```python
from build123d import *

# Parameters (mm, degrees)
BOSS_EXTRUDE1_DEPTH   = 25.4
CUT_EXTRUDE1_REACH    = 329.931
F_8_CLEARANCE_HOLE1_D = 4.9149
CHAMFER1_SIZE         = 1.275307785
CHAMFER1_SIZE_2       = 1.27
CHAMFER1_SIZE_3       = 0.733234842
CUT_EXTRUDE2_DEPTH    = 3.175


with BuildPart() as part:
    # Sketch1 → Boss-Extrude1 (new body)
    with BuildSketch(Plane.XY):
        with BuildLine():
            Line((-288.860017795, -12.750441382), (-326.696640794, -12.750441382))
            ThreePointArc((-326.696640794, -12.750441382), (-307.778329294, -6.400441382), (-288.860017795, -12.750441382))
        make_face()
    extrude(amount=-BOSS_EXTRUDE1_DEPTH)

    # Sketch2 → Cut-Extrude1 (cut, up to next)
    with BuildSketch(Plane.XY, mode=Mode.PRIVATE) as cut_extrude1_sk1:
        with BuildLine():
            Line((-292.035017795, -12.750441382), (-292.035017795, -10.639114407))
            ThreePointArc((-292.035017795, -10.639114407), (-290.415395998, -11.646473343), (-288.860017795, -12.750441382))
            Line((-288.860017795, -12.750441382), (-292.035017795, -12.750441382))
        make_face()
    cut_extrude1_tool1 = extrude(cut_extrude1_sk1.sketch, amount=-CUT_EXTRUDE1_REACH, mode=Mode.PRIVATE) & part.part
    # Sketch2 → Cut-Extrude1 (cut, up to next)
    with BuildSketch(Plane.XY, mode=Mode.PRIVATE) as cut_extrude1_sk2:
        with BuildLine():
            Line((-323.521640794, -12.750441382), (-326.696640794, -12.750441382))
            ThreePointArc((-326.696640794, -12.750441382), (-325.14126259, -11.646473343), (-323.521640794, -10.639114407))
            Line((-323.521640794, -10.639114407), (-323.521640794, -12.750441382))
        make_face()
    cut_extrude1_tool2 = extrude(cut_extrude1_sk2.sketch, amount=-CUT_EXTRUDE1_REACH, mode=Mode.PRIVATE) & part.part
    add(cut_extrude1_tool1.solids().sort_by_distance((-290.95384, -12.03102, 0))[0], mode=Mode.SUBTRACT)
    add(cut_extrude1_tool2.solids().sort_by_distance((-324.602819, -12.03102, 0))[0], mode=Mode.SUBTRACT)

    # #8 Clearance Hole1 (through all)
    with Locations(Plane(origin=(0, -12.750441382, 0), x_dir=(-1, 0, 0), z_dir=(0, -1, 0))):
        with Locations((307.778329294, 12.7)):
            Hole(F_8_CLEARANCE_HOLE1_D / 2)

    # Chamfer1
    # the kernel refuses this chamfer: 1.275307785, 1.27, 0.733234842 mm, written as the material it takes off along each edge
    with BuildSketch(Plane(origin=(-292.035017795, -10.639114407, 3.299478256), x_dir=(-0.8744921081912179, 0.4850397434347821, 0), z_dir=(0, 0, -1))) as chamfer1_piece_1:
        with BuildLine():
            Line((1.228549666, 0), (-CHAMFER1_SIZE * 0.485039743592, -CHAMFER1_SIZE * 0.874492108474))
            Line((-CHAMFER1_SIZE * 0.485039743592, -CHAMFER1_SIZE * 0.874492108474), (0, 0))
            ThreePointArc((0, 0), (0.636104744, 0.006009849), (1.228549666, 0))
        make_face()
    extrude(amount=31.998956511, mode=Mode.SUBTRACT)
    with BuildSketch(Plane(origin=(-323.521640794, -10.639114407, 3.286063629), x_dir=(0.8745288770995413, 0.4849734457875147, 0), z_dir=(0, 0, -1))) as chamfer1_piece_2:
        with BuildLine():
            Line((1.233303065, 0), (-CHAMFER1_SIZE_2 * 0.484973445787, CHAMFER1_SIZE_2 * 0.8745288771))
            Line((-CHAMFER1_SIZE_2 * 0.484973445787, CHAMFER1_SIZE_2 * 0.8745288771), (0, 0))
            ThreePointArc((0, 0), (0.638512102, -0.006056486), (1.233303065, 0))
        make_face()
    extrude(amount=31.972127259, mode=Mode.SUBTRACT)
    # the kernel refuses this chamfer: 1.275307785, 1.27, 0.733234842 mm, written as the material it takes off along each edge
    with BuildSketch(Plane(origin=(-307.778329294, -37.756741382, -25.4), x_dir=(-0.5575773235938082, 0.8301250075825723, 0), z_dir=(-0.8301250075825723, -0.5575773235938082, 0))) as chamfer1_2_piece_1:
        Polygon((31.3563, -CHAMFER1_SIZE_2), (31.3563 - CHAMFER1_SIZE_3, 0), (31.3563, 0), align=None)
    revolve(axis=Axis((-307.778329294, -37.756741382, -25.4), (0, 0, -1)), revolution_arc=67.785524428, mode=Mode.SUBTRACT)
    with BuildSketch(Plane(origin=(-307.778329294, -37.756741382, 0), x_dir=(-0.5575773235938082, 0.8301250075825723, 0), z_dir=(-0.8301250075825723, -0.5575773235938082, 0))) as chamfer1_2_piece_2:
        Polygon((31.3563, CHAMFER1_SIZE_2), (31.3563 - CHAMFER1_SIZE_3, 0), (31.3563, 0), align=None)
    revolve(axis=Axis((-307.778329294, -37.756741382, 0), (0, 0, -1)), revolution_arc=67.785524428, mode=Mode.SUBTRACT)

    # Sketch5 → Cut-Extrude2 (cut)
    with BuildSketch(Plane.XZ.offset(12.750441382)):
        Polygon((-310.417974725, -17.272), (-305.138683864, -17.272), (-302.499038433, -12.7), (-305.138683864, -8.128), (-310.417974725, -8.128), (-313.057620156, -12.7), align=None)
    extrude(amount=-CUT_EXTRUDE2_DEPTH, mode=Mode.SUBTRACT)


solid = part.part
```
The listing builds one solid part. Answer for the finished solid, in the listing's coordinates (mm). A direction names the side the tool comes from. Round coordinates to 2 decimals unless told otherwise and drop trailing zeros. Write each loop counter-clockwise with the first axis right and the second up, starting at its lowest first coordinate (ties: lowest second). Pieces come first, ordered by that corner, then holes. Notation, with made-up numbers: (44, 30) -> (53, 30) arc R15 ccw to (53, 34) -> close; hole circle Ø10 at (60.5, -8). An arc over 180 degrees is marked (long way). Answer as a JSON object with one key per item and string values. Group by question number.
Q1. Each of these flat-tipped pins is pushed along its axis until it touches: pin 1 Ø10 at (x, z) = (-310, -14.5) entering from -Y; pin 2 Ø3 at (x, z) = (-307.78, -12.7) entering from -Y; pin 3 Ø2 at (x, z) = (-320, -20) entering from +Y; pin 4 Ø1.5 at (x, z) = (-318, -9.5) entering from +Y. Where does it stop, or does it pass through?
Q2. Section A-A (z = -7) is taken. Write down the section's boundary in (x, y), plus the area to 3 significant figures.
Q3. Which of the six approach directions +Z, -Z, +X, -X, +Y, -Y give full straight-line access (tool end or side, diameter ignored) to faces 4 (the face through (-322.975, -10.962, -12.522)), 5 (the face through (-311.72, -11.19, -10.38))?
Q4. Straight lines are drawn through the part: line 1 along Z through (x, y) = (-310, -11.5); line 2 along Z through (x, y) = (-311.5, -11); line 3 along X through (y, z) = (-10.5, -15.25). For each, find the intervals that lie inside material, in ascending order.
Q5. Determine the mould class of faces 1 (the face through (-323.522, -12.3, -12.5)), 2 (the face through (-308, -11, 0)), 3 (the face through (-303.8, -11.19, -10.45)) for opening direction X: pulls with the +X half, pulls with the -X half, needs draft (parallel to the pull), parting line crosses it, or undercut.
Check values:
{
 "1": {"pin 1": "y = -12.75", "pin 2": "through", "pin 3": "y = -8.48", "pin 4": "y = -7.87"},
 "2": {"outline": "(-323.52, -12.75) -> (-292.04, -12.75) -> (-292.04, -11.91) -> (-293.11, -10.04) arc R31.36 ccw to (-322.44, -10.04) -> (-323.52, -11.91) -> close", "area": "155 mm^2"},
 "3": {"face 4": "+Z, -Z, -X, +Y", "face 5": "-Y"},
 "4": {"line 1": "-25.4 to -17.27, -8.13 to 0", "line 2": "-25.4 to -15.4, -10 to 0", "line 3": "-322.71 to -311.59, -303.97 to -292.85"},
 "5": {"face 1": "pulls with the -X half", "face 2": "needs draft", "face 3": "undercut"}
}
